Autodesk Inventor part; units mm, degrees
ref_plane "YZ Plane" through (0, 0, 0) normal (1, 0, 0) x (0, 1, 0)
ref_plane "XY Plane" through (0, 0, 0) normal (0, 0, 1) x (1, 0, 0)
sketch "Skizze1" plane through (0, 0, 0) normal (0, 1, 0) x (-1, 0, 0)
  circle A0 centre (0, 0) radius 20
  dimension "d0" = 40
sketch "Skizze2" plane through (0, 0, 0) normal (0, 0, 1) x (1, 0, 0)
  line L0 (0, 0) -> (0, 770)
  line L1 (180, 950) -> (183.4788, 950)
  line L2 (356.6838, 850) -> (680, 290)
  line L3 (680, 290) -> (680, -1250)
  arc A0 (180, 950) -> (0, 770) centre (180, 770) ccw
  arc A1 (356.6838, 850) -> (183.4788, 950) centre (183.4788, 750) ccw
  point P0 (0, 950)
  dimension "d1" = 950
  dimension "d4" = 290
  dimension "d8" = 2200
  dimension "d9" = 30
  dimension "d10" = 680
  dimension "d11" = 180
  dimension "d12" = 200
sweep "Sweeping1" add profiles "Skizze1" path "Skizze2"
sketch "Skizze3" plane through (0, 0, 0) normal (1, 0, 0) x (0, 1, 0)
  circle A0 centre (-20, 0) radius 15
  line L0 (0, 20) -> (0, -20)
  point P0 (0, 0)
  point P1 (0, 0)
  dimension "d16" = 30
  dimension "d27" = 20
extrude "Extrusion1" add sketch "Skizze3" along normal blind 680
sketch "Skizze4" plane through (0, 0, 0) normal (0, -1, 0) x (1, 0, 0)
  circle A0 centre (0, 0) radius 20
extrude "Extrusion2" add sketch "Skizze4" along normal blind 100
ref_plane "Arbeitsebene1" through (0, -20, 0) normal (0, 1, 0) x (-1, 0, 0)
sketch "Skizze5" plane through (0, -20, 0) normal (0, 1, 0) x (-1, 0, 0)
  circle A0 centre (0, 0) radius 20
  circle A1 centre (-500, 0) radius 15
  dimension "d23" = 30
  dimension "d24" = 500
extrude "Extrusion3" add sketch "Skizze5" against normal blind 200 contours A1
ref_plane "Arbeitsebene2" through (500, -160, 0) normal (0, -1, 0) x (1, 0, 0)
sketch "Skizze6" plane through (500, -160, 0) normal (0, -1, 0) x (1, 0, 0)
  circle A0 centre (0, 0) radius 15
  circle A1 centre (180, 0) radius 20
  circle A2 centre (180, 0) radius 20
  circle A3 centre (0, 0) radius 15
  line L0 (0, 15) -> (180, 15)
  line L1 (180, 15) -> (180, -15)
  line L2 (180, -15) -> (0, -15)
  line L3 (0, -15) -> (0, 15)
  point P0 (-500, 0)
  dimension "d29" = 0
  dimension "d30" = 0
  dimension "d31" = 30
  dimension "d32" = 15
extrude "Extrusion4" add sketch "Skizze6" along normal blind 5 contours A0 L3 | A0 L0 A1 L2 | L0 L1 L2 A1 picked at (3.1174, 3.9092) picked at (173.3822, 0.8057)
sketch "Skizze7" plane through (0, -100, 0) normal (0, -1, 0) x (1, 0, 0)
  circle A0 centre (0, 0) radius 20
  circle A1 centre (0, 0) radius 15
  dimension "d35" = 30
extrude "Extrusion5" add sketch "Skizze7" along normal blind 190 contours A1
ref_plane "Arbeitsebene3" through (0, -100, 0) normal (-0.8086, 0, 0.5883) x (0, -1, 0)
sketch "Skizze8" plane through (0, -100, 0) normal (-0.8086, 0, 0.5883) x (0, -1, 0)
  line L0 (190, -15) -> (190, 15)
  line L1 (0, 15) -> (0, -15)
  point P0 (-100, 0)
  point P1 (177.8177, 0)
hole "Bohrung1" at (0, -277.8177, 0) direction (0.8086, 0, -0.5883) diameter 5 end through all both
properties part number "Geländer lang"
The model under review builds one solid part; all positions refer to its coordinate system, in mm. Give positions to 0.01 mm unless a question says otherwise; leave off trailing zeros. Write each loop counter-clockwise with the first axis right and the second up, starting at its lowest first coordinate (ties: lowest second). Pieces come first, ordered by that corner, then holes. Notation, with made-up numbers: M 72,58.5 L 81,58.5 A14 ccw 81,76.5 Z; hole C 14.25,72 d1. An arc over 180 degrees is marked long. One line per question, with ' | ' between items. Start each with the question number.
Item 1: We need section D-D on y = -1004.5. Write out the cut boundary in (x, z), plus the area to 3 significant figures.
Item 2: Wall thickness on line 1 (X direction, y = -114.5, z = 8.5); line 2 (Y direction, x = 531, z = 7.5); line 3 (Y direction, x = 615, z = -12): over which ranges is each line inside the solid? List them lowest first. Write a range as from..to.
Item 3: We need section B-B on z = 0. Give the number of separate pieces and of enclosed holes in the cut face, plus the area to 3 significant figures.
Item 4: We need section A-A on y = 175.5. Write out the cut boundary in (x, z).
Item 5: Draft analysis for pull direction X (two halves, no side actions). For faces 1 (the flat face through (680, -1250, 0)), 2 (the flat face through (3, -100, 15)), state which applies: released by +X, released by -X, zero draft, split by the parting line, or undercut.
Item 6: For pin 1 (9 mm diameter, centred on x = 599.5, z = 3.5, fed in from +Y); pin 2 (1.5 mm diameter, centred on x = 587.5, y = -162.5, fed in from -Z); pin 3 (4 mm diameter, centred on x = 617.5, y = -162, fed in from +Z), all flat-tipped, find the tip position at first contact; note any pin that passes through.
Results found:
1) outline: C 680,0 d40 | area: 1,260 mm2
2) line 1: x = -12.36..12.36, 487.64..512.36, 661.9..698.1 | line 2: y = -165..-160, -32.99..-7.01, 510.99..585.16 | line 3: y = -165..-160, -29..-11, 370.58..434.58
3) separate pieces: 1 | enclosed holes: 3 | area: 173,000 mm2
4) outline: C 0,0 d40; C 680,0 d40
5) face 1: zero draft | face 2: undercut
6) pin 1: stops at y = 476.74 | pin 2: stops at z = -15 | pin 3: stops at z = 15
